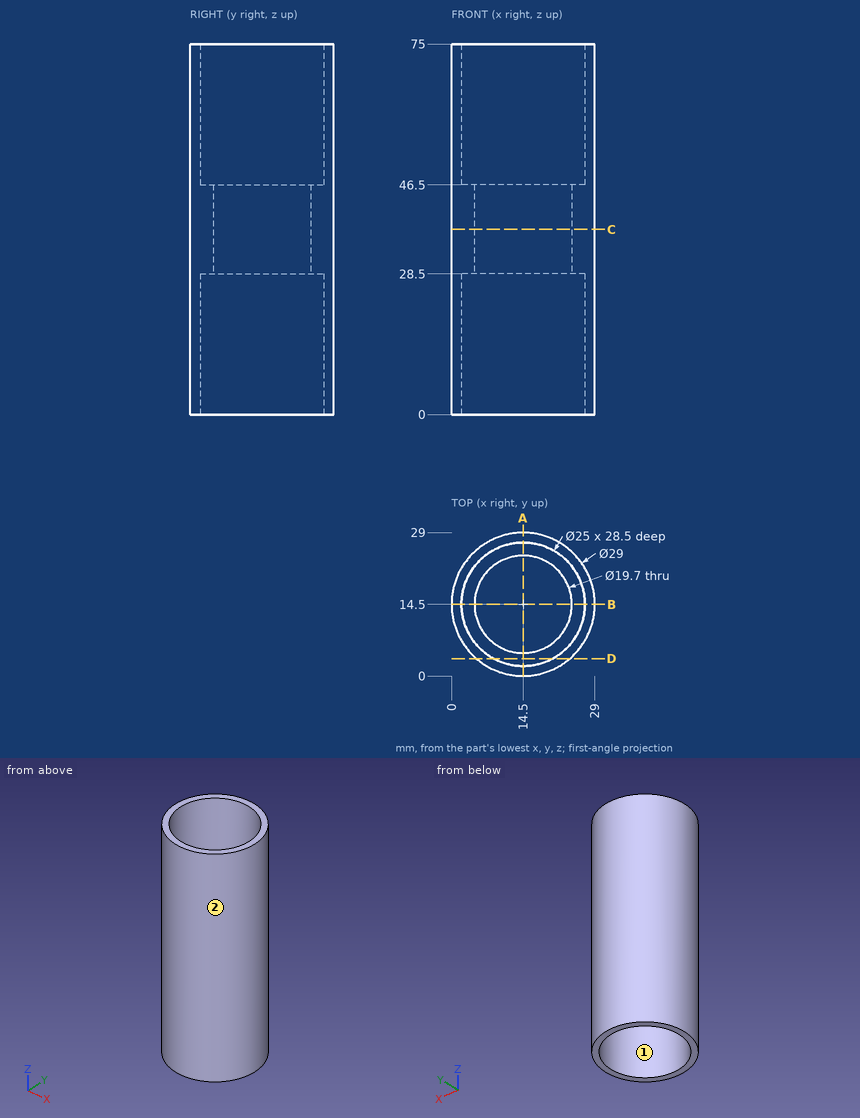
The figure shows three views and two pictorial views of one solid part (mm, origin at its lowest corner). Answer the questions. Round coordinates to 2 decimals unless told otherwise and drop trailing zeros. Write each loop counter-clockwise with the first axis right and the second up, starting at its lowest first coordinate (ties: lowest second). Pieces come first, ordered by that corner, then holes. Notation, with made-up numbers: (68.5, 18) -> (114.5, 18) arc R9 ccw to (114.5, 30) -> close; hole circle Ø5 at (-27, -36.75). An arc over 180 degrees is marked (long way). Answer as a JSON object with one key per item and string values. Group by question number.
Q1. Each of these flat-tipped pins is pushed along its axis until it touches: pin 1 Ø4 at (x, z) = (17, 27) entering from +Y; pin 2 Ø1 at (y, z) = (16, 62.5) entering from +X; pin 3 Ø2 at (x, z) = (4, 52.5) entering from +Y. Where does it stop, or does it pass through?
Q2. Section C-C (z = 37.5) is taken. Write down the section's boundary in (x, y).
Q3. Section A-A (x = 14.5) is taken. Write down the section's boundary in (y, z).
Q4. Determine the mould class of the marked faces 1 and 2 for opening direction X: pulls with the +X half, pulls with the -X half, needs draft (parallel to the pull), parting line crosses it, or undercut.
Q5. Section D-D (y = 3.5) is taken. Write down the section's boundary in (x, z), plus the area to 3 significant figures.
Q6. Straight lines are drawn through the part: line 1 along Y through (x, z) = (14.5, 65.75); line 2 along Y through (x, z) = (14.5, 41); line 3 along Z through (x, y) = (5.5, 6). For each, find the intervals that lie inside material, in ascending order.
Check values:
{
 "1": {"pin 1": "y = 28.99", "pin 2": "x = 28.97", "pin 3": "y = 25.45"},
 "2": {"outline": "circle Ø29 at (14.5, 14.5); hole circle Ø19.7 at (14.5, 14.5)"},
 "3": {"outline": "(0, 0) -> (2, 0) -> (2, 28.5) -> (4.65, 28.5) -> (4.65, 46.5) -> (2, 46.5) -> (2, 75) -> (0, 75) -> close; (24.35, 28.5) -> (27, 28.5) -> (27, 0) -> (29, 0) -> (29, 75) -> (27, 75) -> (27, 46.5) -> (24.35, 46.5) -> close"},
 "4": {"face 1": "undercut", "face 2": "parting line crosses it"},
 "5": {"outline": "(5.05, 0) -> (8.56, 0) -> (8.56, 28.5) -> (20.44, 28.5) -> (20.44, 0) -> (23.95, 0) -> (23.95, 75) -> (20.44, 75) -> (20.44, 46.5) -> (8.56, 46.5) -> (8.56, 75) -> (5.05, 75) -> close", "area": "740 mm^2"},
 "6": {"line 1": "0 to 2, 27 to 29", "line 2": "0 to 4.65, 24.35 to 29", "line 3": "28.5 to 46.5"}
}
